Can you work these out from the drawing? Everything is in mm from the part's minimum corner. A direction names the side the tool comes from. Round coordinates to 2 decimals unless told otherwise and drop trailing zeros. Loops run counter-clockwise (first coordinate to the right, second up) from the corner with the lowest first, then second, coordinate; pieces in that order, holes last. Notation, with made-up numbers: (30, 18.25) -> (38, 18.25) arc R14 cw to (38, 22.25) -> close; hole circle Ø9 at (68, -7.5). An arc over 180 degrees is marked (long way). One line per item, written item: value.
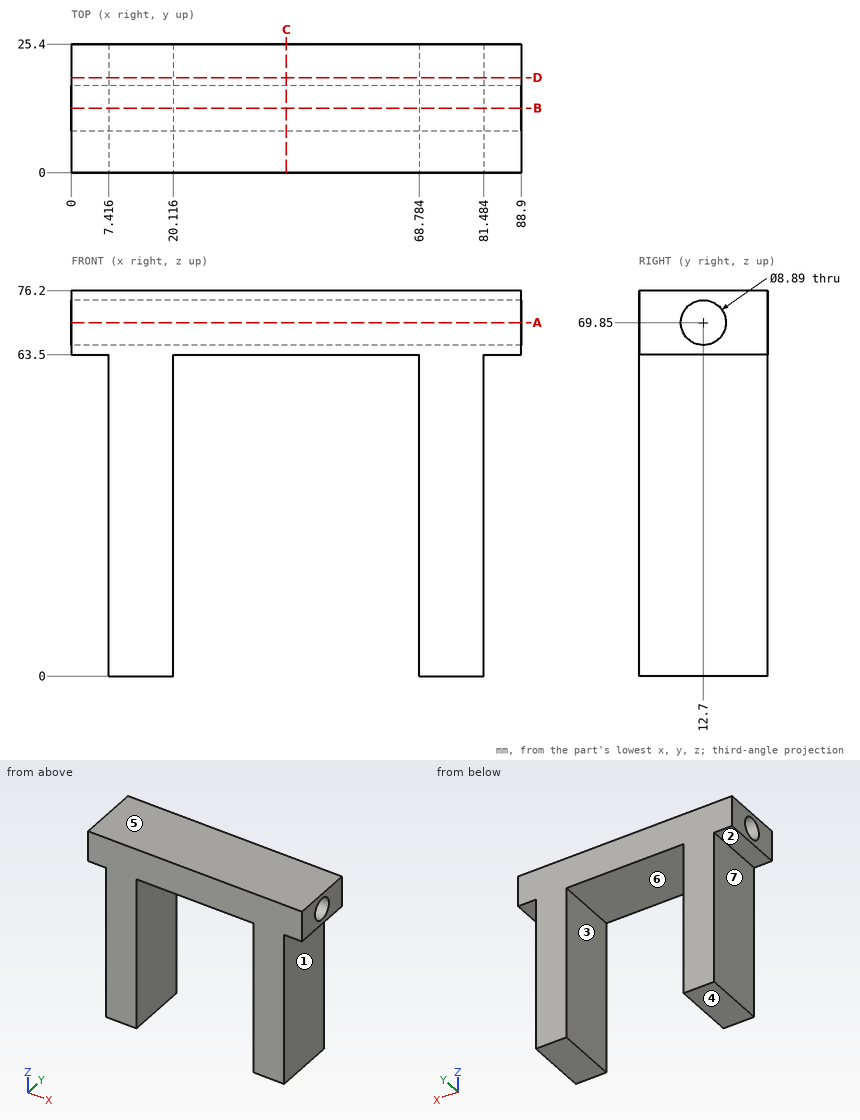
(1) If we section it at B-B, the plane y = 12.7: Please give me the cut outline in (x, z) (3 decimals), then the cut area to 3 significant figures.
Recorded:
outline: (0, 63.5) -> (7.416, 63.5) -> (7.416, 0) -> (20.116, 0) -> (20.116, 63.5) -> (68.784, 63.5) -> (68.784, 0) -> (81.484, 0) -> (81.484, 63.5) -> (88.9, 63.5) -> (88.9, 65.405) -> (0, 65.405) -> close; (0, 74.295) -> (88.9, 74.295) -> (88.9, 76.2) -> (0, 76.2) -> close
area: 1,950 mm²
(2) I'm going to push flat-ended pins straight in: pin 1 Ø12.5 at (y, z) = (10, 33) entering from +X; pin 2 Ø4 at (y, z) = (8, 21) entering from -X; pin 3 Ø12 at (x, z) = (14, 27.5) entering from -Y; pin 4 Ø6 at (x, y) = (4, 19) entering from -Z. Where does each tip first touch, or does it pass through?
Recorded:
pin 1: x = 81.48
pin 2: x = 7.42
pin 3: y = 0
pin 4: z = 63.5
(3) Thinking about a two-plate mould opening in X: for the marked faces 5, 6 and 7, which applies, released by +X, released by -X, zero draft, split by the parting line, or undercut?
Recorded:
face 5: zero draft
face 6: undercut
face 7: released by -X
(4) If I drill on L1, parallel to X at y = 11.25, z = 34.5; L2, parallel to Z at x = 22.5, y = 12.7 (3 decimals); L3, parallel to Y at x = 19, z = 69, over which ranges is the centre line in solid material (lowest first)?
Recorded:
L1: 7.42 to 20.12, 68.78 to 81.48
L2: 63.5 to 65.405, 74.295 to 76.2
L3: 0 to 8.34, 17.06 to 25.4
(5) If we section it at C-C, the plane x = 42.5: Please give me the cut outline in (y, z) (3 decimals).
Recorded:
outline: (0, 63.5) -> (25.4, 63.5) -> (25.4, 76.2) -> (0, 76.2) -> close; hole circle Ø8.89 at (12.7, 69.85)
(6) If we section it at D-D, the plane y = 18.75: Please give me the cut outline in (x, z), then the cut area to 3 significant figures.
Recorded:
outline: (0, 63.5) -> (7.42, 63.5) -> (7.42, 0) -> (20.12, 0) -> (20.12, 63.5) -> (68.78, 63.5) -> (68.78, 0) -> (81.48, 0) -> (81.48, 63.5) -> (88.9, 63.5) -> (88.9, 76.2) -> (0, 76.2) -> close
area: 2,740 mm²
(7) For the marked faces 1, 2, 3 and 4, which set-ups out of +Z, -Z, +X, -X, +Y, -Y let a thin tool reach every point of the face, with its end or its side?
Recorded:
face 1: -Z, +X, +Y, -Y
face 2: -Z, -X, +Y, -Y
face 3: -Z, +Y, -Y
face 4: -Z, +X, -X, +Y, -Y
(8) If we section it at A-A, the plane z = 69.85: Please give me the cut outline in (x, y) (3 decimals), then the cut area to 3 significant figures.
Recorded:
outline: (0, 0) -> (88.9, 0) -> (88.9, 8.255) -> (0, 8.255) -> close; (0, 17.145) -> (88.9, 17.145) -> (88.9, 25.4) -> (0, 25.4) -> close
area: 1,470 mm²
